from build123d import *

# Parameters (mm, degrees)
F0_W      = 135.5
F0_H      = 82
F0_R      = 35.5
F1_DEPTH  = 1
F2_R      = 36
F4_R      = 23
F6_W      = 135.5
F6_H      = 82
F6_W_2    = 133.5
F6_H_2    = 80
F7_DEPTH  = 25
F8_R      = 15
F9_DEPTH  = 17
F11_DEPTH = 17
F12_W     = 26
F12_H     = 135.5
F13_DEPTH = 1
F14_W     = 8.678573
F14_H     = 5.408388
F14_W_2   = 10.062111
F15_DEPTH = 17.4


with BuildPart() as f1:
    # F0 (on Right) → F1 (new body)
    with BuildSketch(Plane.YZ):
        Rectangle(F0_W, F0_H)
        Circle(F0_R, mode=Mode.SUBTRACT)
    extrude(amount=F1_DEPTH)

    # F2 (on face) → F5 section 0
    with BuildSketch(Plane(origin=(0, 0, 0), x_dir=(0, -1, 0), z_dir=(-1, 0, 0))):
        Circle(F2_R)
    # F4 (on offset) → F5 section 1
    with BuildSketch(Plane.YZ.offset(-53)):
        Circle(F4_R)
    loft()

    # F6 (on face) → F7 (join)
    with BuildSketch(Plane.YZ.offset(1)):
        Rectangle(F6_W, F6_H)
        Rectangle(F6_W_2, F6_H_2, mode=Mode.SUBTRACT)
    extrude(amount=F7_DEPTH)

    # F8 (on face) → F9 (join)
    with BuildSketch(Plane.XY.offset(41)):
        with Locations((13, 52.75)):
            Circle(F8_R)
    extrude(amount=F9_DEPTH)

    # F10 (on face) → F11 (join)
    with BuildSketch(Plane.XY.offset(41)):
        with BuildLine():
            Line((0, -67.75), (26, -67.75))
            Line((26, -67.75), (26, 45.266685))
            ThreePointArc((26, 45.266685), (13, 37.770541), (0, 45.266685))
            Line((0, 45.266685), (0, -67.75))
        make_face()
        with BuildLine():
            Line((24.066526, -66.408634), (1.175221, -66.408634))
            Line((1.175221, -66.408634), (1.175221, 40.501304))
            ThreePointArc((1.175221, 40.501304), (12.523338, 35.811878), (24.066526, 39.9982))
            Line((24.066526, 39.9982), (24.066526, -66.408634))
        make_face(mode=Mode.SUBTRACT)
    extrude(amount=F11_DEPTH)

    # F12 (on face) → F13 (join)
    with BuildSketch(Plane.XY.offset(58)):
        with Locations((13, 0)):
            Rectangle(F12_W, F12_H)
    extrude(amount=F13_DEPTH)

    # F14 (on face) → F15 (cut)
    with BuildSketch(Plane(origin=(0, 0, 0), x_dir=(0, -1, 0), z_dir=(-1, 0, 0))):
        with Locations((22.075063, 50.707543)):
            Rectangle(F14_W, F14_H)
        with Locations((-14.84031, 50.707543)):
            Rectangle(F14_W_2, F14_H)
    extrude(amount=-F15_DEPTH, mode=Mode.SUBTRACT)


solid = f1.part
Can you work these out from the model? Positions are in its coordinate system, mm. A direction names the side the tool comes from. Round coordinates to 2 decimals unless told otherwise and drop trailing zeros. Order: outer loops, then holes, each group sorted by start corner. A loop starts at its lowest first (then second) coordinate and runs counter-clockwise, first axis right, second up. Notation, with made-up numbers: (0.25, -37.75) -> (58.25, -37.75) arc R35 ccw to (58.25, -4.75) -> close; hole circle Ø2 at (80.25, 38). An arc over 180 degrees is marked (long way). Write each question's results on one line, items separated by ' | '. Start each with the question number.
Item 1: If we section it at A-A, the plane z = 50.5: Write out the boundary of the cut face in (x, y).
Item 2: If we section it at D-D, the plane y = 52.75: Write out the boundary of the cut face in (x, z).
Item 3: Thinking about a two-plate mould opening in X: for faces 4 (the flat face through (13, 1, 59)), 5 (the cylindrical face through (13.439, 67.744, 49.381)), 6 (the flat face through (1, -31, 18)), 7 (the flat face through (1.175, -14, 49)), which applies, +X half, -X half, draft (parallel to the pull), parting line (faces both ways), or undercut?
Item 4: Will these pins go through, and if not, where does the flat tip stop? pin 1 (0.6 mm diameter, centred on x = 26.5, y = 50, fed in from +Z); pin 2 (1.5 mm diameter, centred on x = -19.5, z = 16, fed in from -Y); pin 3 (4 mm diameter, centred on y = -37.5, z = 16, fed in from +X).
Item 5: If we section it at C-C, the plane x = 20: Write out the boundary of the cut face in (y, z).
Item 6: Which directions (+Z, -Z, +X, -X, +Y, -Y) give clear straight access to the entire face, cutting with the end or side of a thin tool? Please do faces 1 (the flat face through (3, 66, 58)), 2 (the cylindrical face through (0.493, -7.696, -34.656)), 3 (the flat face through (13, -66.409, 49)).
Item 7: Please list where these lines run through material, in increasing order: L1, parallel to Z at x = 8, y = -42.5; L2, parallel to Y at x = 2, z = -14.5; L3, parallel to X at y = 7, z = 44.5.
Item 8: If we section it at B-B, the plane y = -55: Write out the boundary of the cut face in (x, z), then the cut area to 3 significant figures.
Results:
1) outline: (0, -67.75) -> (26, -67.75) -> (26, 45.27) arc R15 ccw (long way) to (0, 45.27) -> (0, 19.87) -> (1.18, 19.87) -> (1.18, 40.5) arc R16.98 ccw to (24.07, 40) -> (24.07, -66.41) -> (1.18, -66.41) -> (1.18, -26.41) -> (0, -26.41) -> close; (0, -17.74) -> (1.18, -17.74) -> (1.18, 9.81) -> (0, 9.81) -> close
2) outline: (-2, 41) -> (0, 41) -> (0, -41) -> (26, -41) -> (26, -40) -> (1, -40) -> (1, 40) -> (26, 40) -> (26, 41) -> (28, 41) -> (28, 58) -> (26, 58) -> (26, 59) -> (0, 59) -> (0, 58) -> (-2, 58) -> close
3) face 4: draft | face 5: parting line | face 6: +X half | face 7: undercut
4) pin 1: stops at z = 58 | pin 2: stops at y = -27.29 | pin 3: stops at x = 1
5) outline: (-67.75, -41) -> (67.75, -41) -> (67.75, 41) -> (66.02, 41) -> (66.02, 58) -> (67.75, 58) -> (67.75, 59) -> (-67.75, 59) -> close; hole (-66.75, -40) -> (66.75, -40) -> (66.75, 40) -> (-66.75, 40) -> close; hole (-66.41, 41) -> (37.36, 41) -> (37.36, 58) -> (-66.41, 58) -> close
6) face 1: -X, +Y | face 2: +X | face 3: none
7) L1: z = -41 to -40, 40 to 41, 58 to 59 | L2: y = -67.75 to -66.75, 66.75 to 67.75 | L3: x = 0 to 1.18, 24.07 to 26
8) outline: (0, -41) -> (26, -41) -> (26, -40) -> (1, -40) -> (1, 40) -> (26, 40) -> (26, 59) -> (0, 59) -> close; hole (1.18, 41) -> (24.07, 41) -> (24.07, 58) -> (1.18, 58) -> close | area: 211 mm2
